Design review of the part built by this model. Coordinates are the model's own, in mm. A direction names the side the tool comes from. Coordinates: 2 decimals unless noted, no trailing zeros. Write each loop counter-clockwise with the first axis right and the second up, starting at its lowest first coordinate (ties: lowest second). Pieces come first, ordered by that corner, then holes.
Q1. The part is to be moulded in two halves that separate along X. For faces 1 (the flat face through (-1.905, 0, -65)), 2 (the flat face through (175.895, 0, -65)), 3 (the flat face through (177.773, 9.514, -62.159)), say which applies: released by +X, released by -X, zero draft, split by the parting line, or undercut.
Q2. For faces 4 (the flat face through (177.8, 0, 4)), 5 (the flat face through (177.773, -9.514, -62.159)), 6 (the flat face through (88, 0, -63.5)), 7 (the flat face through (0, 0, 4)), 8 (the flat face through (88, -3.175, 17)), list the 3-axis set-ups (+Z, -Z, +X, -X, +Y, -Y) from which the entire face can be reached by the end or side of a thin tool; tool diameter is ignored.
Q3. For pin 1 Ø6 at (x, y) = (112, -5.5) entering from -Z; pin 2 Ø1.6 at (x, y) = (86.5, -5) entering from +Z (3 decimals); pin 3 Ø6 at (x, z) = (58, 9.5) entering from -Y (3 decimals); pin 4 Ø10 at (x, y) = (69.5, 11.5) entering from +Z, all flat-tipped, find the tip position at first contact; note any pin that passes through.
Q4. Take a section at C-C, the plane z = -24.5. Write out the cut boundary in (x, y) (3 decimals).
Q5. Take a section at A-A, the plane x = 31.5. Write out the cut boundary in (y, z) (3 decimals), plus the area to 3 significant figures.
Q6. For L1, parallel to Y at x = 163, z = 17.5 (3 decimals); L2, parallel to Z at x = 138, y = 3; L3, parallel to Z at x = 53.5, y = -4 (3 decimals), list the stretches that pass through material, from the lowest coordinate up.
Q7. Take a section at B-B, the plane y = -10.5. Write out the cut boundary in (x, z) (3 decimals).
from build123d import *

# Parameters (mm, degrees)
F0_W          = 6.35
F0_H          = 127
F1_DEPTH      = 177.8
F2_W          = 3.81
F2_H          = 12.7
F3_DEPTH      = 12.7
F3_DEPTH_BACK = 19.05
F4_SIZE2      = 12.5465551104
F4_SIZE       = 10.16
F4_2_SIZE2    = 12.5465551104
F4_2_SIZE     = 10.16
F4_3_SIZE2    = 12.5465551104
F4_3_SIZE     = 10.16
F5_SIZE2      = 12.5465551104
F5_SIZE       = 10.16
F7_DEPTH      = 177.8


with BuildPart() as f1:
    # F0 (on Right) → F1 (new body)
    with BuildSketch(Plane.YZ):
        Rectangle(F0_W, F0_H)
    extrude(amount=F1_DEPTH)

    # F2 (on face) → F3 (join, two sides)
    with BuildSketch(Plane.XZ.offset(3.175)) as f3_sk:
        with Locations((0, -63.5)):
            Rectangle(F2_W, F2_H)
        with Locations((177.8, -63.5)):
            Rectangle(F2_W, F2_H)
    extrude(amount=F3_DEPTH)
    extrude(f3_sk.sketch, amount=-F3_DEPTH_BACK)

    # F4
    f4_edges = [f1.edges().sort_by_distance(p)[0] for p in [
        (177.8, -15.875, -57.15),
    ]]
    f4_side = f1.faces().sort_by_distance((177.8, -15.875, -63.5))[0]
    chamfer(f4_edges, length=F4_SIZE, length2=F4_SIZE2, reference=f4_side)

    # F4#2
    f4_2_edges = [f1.edges().sort_by_distance(p)[0] for p in [
        (177.8, 15.875, -57.15),
    ]]
    f4_2_side = f1.faces().sort_by_distance((177.8, 15.875, -63.5))[0]
    chamfer(f4_2_edges, length=F4_2_SIZE, length2=F4_2_SIZE2, reference=f4_2_side)

    # F4#3
    f4_3_edges = [f1.edges().sort_by_distance(p)[0] for p in [
        (0, -15.875, -57.15),
    ]]
    f4_3_side = f1.faces().sort_by_distance((0, -15.875, -63.5))[0]
    chamfer(f4_3_edges, length=F4_3_SIZE, length2=F4_3_SIZE2, reference=f4_3_side)

    # F5
    f5_edges = [f1.edges().sort_by_distance(p)[0] for p in [
        (0, 15.875, -57.15),
    ]]
    f5_side = f1.faces().sort_by_distance((0, 15.875, -63.5))[0]
    chamfer(f5_edges, length=F5_SIZE, length2=F5_SIZE2, reference=f5_side)

    # F6 (on face) → F7 (join)
    with BuildSketch(Plane.YZ.offset(177.8)):
        Polygon((6.35, -27.305), (0, -27.305), (0, -28.575), (0, -29.845), (6.35, -29.845), align=None)
        Polygon((0, -28.575), (0, -27.305), (-6.35, -27.305), (-6.35, -29.845), (0, -29.845), align=None)
    extrude(amount=-F7_DEPTH)


solid = f1.part
Responses:
1. face 1: released by -X
1. face 2: undercut
1. face 3: zero draft
2. face 4: +Z, +X, +Y, -Y
2. face 5: +X, -X, -Y
2. face 6: -Z, +Y, -Y
2. face 7: +Z, -X, +Y, -Y
2. face 8: +Z, +X, -X, -Y
3. pin 1: stops at z = -63.5
3. pin 2: stops at z = -27.305
3. pin 3: stops at y = -3.175
3. pin 4: passes through
4. outline: (0, -3.175) - (177.8, -3.175) - (177.8, 3.175) - (0, 3.175) - close
5. outline: (-6.35, -29.845) - (-3.175, -29.845) - (-3.175, -63.5) - (3.175, -63.5) - (3.175, -29.845) - (6.35, -29.845) - (6.35, -27.305) - (3.175, -27.305) - (3.175, 63.5) - (-3.175, 63.5) - (-3.175, -27.305) - (-6.35, -27.305) - close
5. area: 823 mm2
6. L1: y = -3.175 to 3.175
6. L2: z = -63.5 to 63.5
6. L3: z = -29.845 to -27.305
7. outline: (-1.905, -69.85) - (1.905, -69.85) - (1.905, -62.957) - (-1.905, -62.957) - close; (175.895, -69.85) - (179.705, -69.85) - (179.705, -62.957) - (175.895, -62.957) - close
